Part model, mm, in its own coordinate system. Face numbers are marked on the shaded views. Round coordinates to 2 decimals unless told otherwise and drop trailing zeros. Loops run counter-clockwise (first coordinate to the right, second up) from the corner with the lowest first, then second, coordinate; pieces in that order, holes last. Notation, with made-up numbers: M -39.75,62 L 17.25,62 A29 cw 17.25,99 Z; hole C 20.25,71.5 d7. An arc over 180 degrees is marked long. Answer as CSV lines item,"result". Start each with the question number.
Item 1: Drop flat-ended pins along their axis: pin 1 Ø1.6 at (y, z) = (3, 2.5) entering from -X; pin 2 Ø5 at (x, y) = (22, 5) entering from +Z; pin 3 Ø1.6 at (x, z) = (4.5, 2.5) entering from +Y; pin 4 Ø1.2 at (x, z) = (21.5, 2.5) entering from -Y. Give the stop position or say it passes through.
Item 2: Band-saw the part on A-A (x = 29.5). Give the cut face in (y, z).
Item 3: Wall check: line 1 (Y direction, x = 52.2, z = 0.6); line 2 (Z direction, x = 19, y = 11.5); line 3 (Y direction, x = 53, z = 0.5). Give the ranges that are in metal, low to high.
Item 4: Mould opens along X. For the marked faces 1 and 2 say: pulls with the +X half, pulls with the -X half, needs draft (parallel to the pull), parting line crosses it, or undercut.
```python
from build123d import *

# Parameters (mm, degrees)
ESBO_O1_W                = 67
ESBO_O1_H                = 17
RESSALTO_EXTRUS_O1_DEPTH = 1.6
ESBO_O2_R                = 1.55
CORTE_EXTRUS_O1_DEPTH    = 70.141593849
ESBO_O3_W                = 2.7
ESBO_O3_H                = 3.4
RESSALTO_EXTRUS_O2_DEPTH = 1.5


with BuildPart() as part:
    # Esboço1 → Ressalto-extrusão1 (new body)
    with BuildSketch(Plane.XY):
        with Locations((33.5, 8.5)):
            Rectangle(ESBO_O1_W, ESBO_O1_H)
    extrude(amount=RESSALTO_EXTRUS_O1_DEPTH)

    # Esboço2 → Corte-extrusão1 (cut, through all)
    with BuildSketch(Plane.XY.offset(1.6)):
        with Locations((14.8, 13.25)):
            Circle(ESBO_O2_R)
        with Locations((52.2, 13.25)):
            Circle(ESBO_O2_R)
    extrude(amount=-CORTE_EXTRUS_O1_DEPTH, mode=Mode.SUBTRACT)

    # Esboço3 → Ressalto-extrusão2 (add)
    with BuildSketch(Plane.XY.offset(1.6)):
        with Locations((5.15, 2.7)):
            Rectangle(ESBO_O3_W, ESBO_O3_H)
        with Locations((13.25, 2.7)):
            Rectangle(ESBO_O3_W, ESBO_O3_H)
        with Locations((21.35, 2.7)):
            Rectangle(ESBO_O3_W, ESBO_O3_H)
        with Locations((29.45, 2.7)):
            Rectangle(ESBO_O3_W, ESBO_O3_H)
        with Locations((37.55, 2.7)):
            Rectangle(ESBO_O3_W, ESBO_O3_H)
        with Locations((45.65, 2.7)):
            Rectangle(ESBO_O3_W, ESBO_O3_H)
        with Locations((53.75, 2.7)):
            Rectangle(ESBO_O3_W, ESBO_O3_H)
        with Locations((61.85, 2.7)):
            Rectangle(ESBO_O3_W, ESBO_O3_H)
    extrude(amount=RESSALTO_EXTRUS_O2_DEPTH)


solid = part.part
```
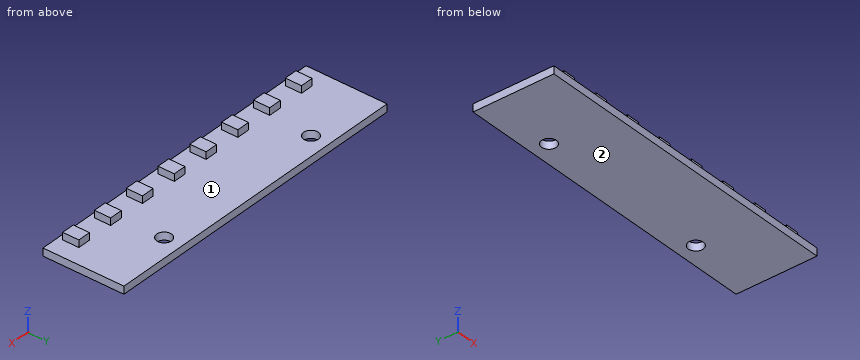
Answer block:
1,pin 1,"stops at x = 3.8"
1,pin 2,"stops at z = 3.1"
1,pin 3,"stops at y = 4.4"
1,pin 4,"stops at y = 1"
2,outline,"M 0,0 L 17,0 L 17,1.6 L 4.4,1.6 L 4.4,3.1 L 1,3.1 L 1,1.6 L 0,1.6 Z"
3,line 1,"y = 0 to 11.7, 14.8 to 17"
3,line 2,"z = 0 to 1.6"
3,line 3,"y = 0 to 11.92, 14.58 to 17"
4,face 1,"undercut"
4,face 2,"needs draft"
